Geometry: final body of the model. Coordinates: model frame, mm. Face numbers are marked on the shaded views. A direction names the side the tool comes from. Round coordinates to 2 decimals unless told otherwise and drop trailing zeros. Loops run counter-clockwise (first coordinate to the right, second up) from the corner with the lowest first, then second, coordinate; pieces in that order, holes last. Notation, with made-up numbers: (31, 85) -> (52, 85) arc R21 ccw to (52, 111) -> close; hole circle Ø7 at (71, -23.5). An arc over 180 degrees is marked (long way). Answer in a Markdown table with one row per item.
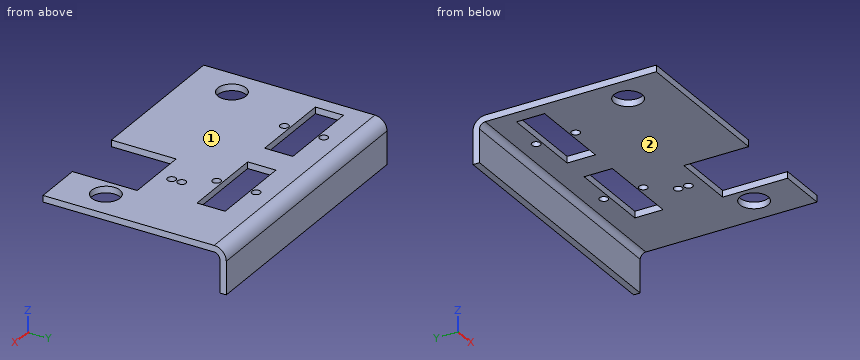
```python
from build123d import *

# Parameters (mm, degrees)
SKETCH1_W                    = 95
SKETCH1_H                    = 65
BASE_FLANGE1_DEPTH           = 2.3
EDGE_FLANGE1_STRIP_W         = 13.2
EDGE_FLANGE1_STRIP_H         = 2.3
EDGE_FLANGE1_STRIP_CUT_DEPTH = 95
EDGE_FLANGE1_DEPTH           = 95
CUT_EXTRUDE1_REACH           = 118.215
SKETCH9_R                    = 1.5
SKETCH9_W                    = 23
SKETCH9_H                    = 23
CUT_EXTRUDE3_REACH           = 117.921
SKETCH10_R                   = 1.5
SKETCH10_W                   = 30
SKETCH10_H                   = 10
CUT_EXTRUDE4_REACH           = 117.921
SKETCH11_R                   = 5


# Sheet-metal steps are written as plain solids
with BuildPart() as part:
    # Sketch1 → Base-Flange1 (new body)
    with BuildSketch(Plane.XY):
        with Locations((47.5, 32.5)):
            Rectangle(SKETCH1_W, SKETCH1_H)
    extrude(amount=-BASE_FLANGE1_DEPTH)

    # Edge-Flange1 strip (across the edge) → Edge-Flange1 strip cut (cut)
    with BuildSketch(Plane(origin=(0, 65, -2.3), x_dir=(0, -1, 0), z_dir=(1, 0, 0))):
        with Locations((-2.3, -1.15)):
            Rectangle(EDGE_FLANGE1_STRIP_W, EDGE_FLANGE1_STRIP_H)
    extrude(amount=EDGE_FLANGE1_STRIP_CUT_DEPTH, mode=Mode.SUBTRACT)

    # Edge-Flange1 section (across the edge) → Edge-Flange1 (add)
    with BuildSketch(Plane(origin=(0, 65, -2.3), x_dir=(0, -1, 0), z_dir=(1, 0, 0))):
        with BuildLine():
            Line((0, 2), (0, 13.7))
            Line((0, 13.7), (2.3, 13.7))
            Line((2.3, 13.7), (2.3, 2))
            ThreePointArc((2.3, 2), (2.885786438, 0.585786438), (4.3, 0))
            Line((4.3, 0), (4.3, -2.3))
            ThreePointArc((4.3, -2.3), (1.259440841, -1.040559159), (0, 2))
        make_face()
    extrude(amount=EDGE_FLANGE1_DEPTH)

    # Sketch9 → Cut-Extrude1 (cut, up to next)
    with BuildSketch(Plane.XY, mode=Mode.PRIVATE) as cut_extrude1_sk1:
        with Locations((66.12, 28.3)):
            Circle(SKETCH9_R)
    cut_extrude1_tool1 = extrude(cut_extrude1_sk1.sketch, amount=-CUT_EXTRUDE1_REACH, mode=Mode.PRIVATE) & part.part
    # Sketch9 → Cut-Extrude1 (cut, up to next)
    with BuildSketch(Plane.XY, mode=Mode.PRIVATE) as cut_extrude1_sk2:
        with Locations((66.12, 31.9)):
            Circle(SKETCH9_R)
    cut_extrude1_tool2 = extrude(cut_extrude1_sk2.sketch, amount=-CUT_EXTRUDE1_REACH, mode=Mode.PRIVATE) & part.part
    # Sketch9 → Cut-Extrude1 (cut, up to next)
    with BuildSketch(Plane.XY, mode=Mode.PRIVATE) as cut_extrude1_sk3:
        with Locations((66.12, 11.5)):
            Rectangle(SKETCH9_W, SKETCH9_H)
    cut_extrude1_tool3 = extrude(cut_extrude1_sk3.sketch, amount=-CUT_EXTRUDE1_REACH, mode=Mode.PRIVATE) & part.part
    add(cut_extrude1_tool1.solids().sort_by_distance((66.12, 28.3, 0))[0], mode=Mode.SUBTRACT)
    add(cut_extrude1_tool2.solids().sort_by_distance((66.12, 31.9, 0))[0], mode=Mode.SUBTRACT)
    add(cut_extrude1_tool3.solids().sort_by_distance((66.12, 11.5, 0))[0], mode=Mode.SUBTRACT)

    # Sketch10 → Cut-Extrude3 (cut, up to next)
    with BuildSketch(Plane(origin=(0, 0, -2.3), x_dir=(-1, 0, 0), z_dir=(0, 0, -1)), mode=Mode.PRIVATE) as cut_extrude3_sk1:
        with Locations((-60, 54.6)):
            Circle(SKETCH10_R)
    cut_extrude3_tool1 = extrude(cut_extrude3_sk1.sketch, amount=-CUT_EXTRUDE3_REACH, mode=Mode.PRIVATE) & part.part
    # Sketch10 → Cut-Extrude3 (cut, up to next)
    with BuildSketch(Plane(origin=(0, 0, -2.3), x_dir=(-1, 0, 0), z_dir=(0, 0, -1)), mode=Mode.PRIVATE) as cut_extrude3_sk2:
        with Locations((-60, 40.6)):
            Circle(SKETCH10_R)
    cut_extrude3_tool2 = extrude(cut_extrude3_sk2.sketch, amount=-CUT_EXTRUDE3_REACH, mode=Mode.PRIVATE) & part.part
    # Sketch10 → Cut-Extrude3 (cut, up to next)
    with BuildSketch(Plane(origin=(0, 0, -2.3), x_dir=(-1, 0, 0), z_dir=(0, 0, -1)), mode=Mode.PRIVATE) as cut_extrude3_sk3:
        with Locations((-20, 54.6)):
            Circle(SKETCH10_R)
    cut_extrude3_tool3 = extrude(cut_extrude3_sk3.sketch, amount=-CUT_EXTRUDE3_REACH, mode=Mode.PRIVATE) & part.part
    # Sketch10 → Cut-Extrude3 (cut, up to next)
    with BuildSketch(Plane(origin=(0, 0, -2.3), x_dir=(-1, 0, 0), z_dir=(0, 0, -1)), mode=Mode.PRIVATE) as cut_extrude3_sk4:
        with Locations((-20, 40.6)):
            Circle(SKETCH10_R)
    cut_extrude3_tool4 = extrude(cut_extrude3_sk4.sketch, amount=-CUT_EXTRUDE3_REACH, mode=Mode.PRIVATE) & part.part
    # Sketch10 → Cut-Extrude3 (cut, up to next)
    with BuildSketch(Plane(origin=(0, 0, -2.3), x_dir=(-1, 0, 0), z_dir=(0, 0, -1)), mode=Mode.PRIVATE) as cut_extrude3_sk5:
        with Locations((-20, 47.6)):
            Rectangle(SKETCH10_W, SKETCH10_H)
    cut_extrude3_tool5 = extrude(cut_extrude3_sk5.sketch, amount=-CUT_EXTRUDE3_REACH, mode=Mode.PRIVATE) & part.part
    # Sketch10 → Cut-Extrude3 (cut, up to next)
    with BuildSketch(Plane(origin=(0, 0, -2.3), x_dir=(-1, 0, 0), z_dir=(0, 0, -1)), mode=Mode.PRIVATE) as cut_extrude3_sk6:
        with Locations((-60, 47.6)):
            Rectangle(SKETCH10_W, SKETCH10_H)
    cut_extrude3_tool6 = extrude(cut_extrude3_sk6.sketch, amount=-CUT_EXTRUDE3_REACH, mode=Mode.PRIVATE) & part.part
    add(cut_extrude3_tool1.solids().sort_by_distance((60, 54.6, -2.3))[0], mode=Mode.SUBTRACT)
    add(cut_extrude3_tool2.solids().sort_by_distance((60, 40.6, -2.3))[0], mode=Mode.SUBTRACT)
    add(cut_extrude3_tool3.solids().sort_by_distance((20, 54.6, -2.3))[0], mode=Mode.SUBTRACT)
    add(cut_extrude3_tool4.solids().sort_by_distance((20, 40.6, -2.3))[0], mode=Mode.SUBTRACT)
    add(cut_extrude3_tool5.solids().sort_by_distance((20, 47.6, -2.3))[0], mode=Mode.SUBTRACT)
    add(cut_extrude3_tool6.solids().sort_by_distance((60, 47.6, -2.3))[0], mode=Mode.SUBTRACT)

    # Sketch11 → Cut-Extrude4 (cut, up to next)
    with BuildSketch(Plane(origin=(0, 0, -2.3), x_dir=(-1, 0, 0), z_dir=(0, 0, -1)), mode=Mode.PRIVATE) as cut_extrude4_sk1:
        with Locations((-10, 16)):
            Circle(SKETCH11_R)
    cut_extrude4_tool1 = extrude(cut_extrude4_sk1.sketch, amount=-CUT_EXTRUDE4_REACH, mode=Mode.PRIVATE) & part.part
    # Sketch11 → Cut-Extrude4 (cut, up to next)
    with BuildSketch(Plane(origin=(0, 0, -2.3), x_dir=(-1, 0, 0), z_dir=(0, 0, -1)), mode=Mode.PRIVATE) as cut_extrude4_sk2:
        with Locations((-84.5, 16)):
            Circle(SKETCH11_R)
    cut_extrude4_tool2 = extrude(cut_extrude4_sk2.sketch, amount=-CUT_EXTRUDE4_REACH, mode=Mode.PRIVATE) & part.part
    add(cut_extrude4_tool1.solids().sort_by_distance((10, 16, -2.3))[0], mode=Mode.SUBTRACT)
    add(cut_extrude4_tool2.solids().sort_by_distance((84.5, 16, -2.3))[0], mode=Mode.SUBTRACT)


solid = part.part
```
Item 1: Section query B-B, the plane y = 54.6. Output: boundary loops of the cut face in (x, z), and give its area (3 significant figures).
Ans:
| item | result |
|---|---|
| outline | (0, -2.3) -> (18.5, -2.3) -> (18.5, 0) -> (0, 0) -> close; (21.5, -2.3) -> (58.5, -2.3) -> (58.5, 0) -> (21.5, 0) -> close; (61.5, -2.3) -> (95, -2.3) -> (95, 0) -> (61.5, 0) -> close |
| area | 205 mm2 |
Item 2: Section query D-D, the plane y = 16. Output: boundary loops of the cut face in (x, z), and give its area (3 significant figures).
Ans:
| item | result |
|---|---|
| outline | (0, -2.3) -> (5, -2.3) -> (5, 0) -> (0, 0) -> close; (15, -2.3) -> (54.62, -2.3) -> (54.62, 0) -> (15, 0) -> close; (77.62, -2.3) -> (79.5, -2.3) -> (79.5, 0) -> (77.62, 0) -> close; (89.5, -2.3) -> (95, -2.3) -> (95, 0) -> (89.5, 0) -> close |
| area | 120 mm2 |
Item 3: First-contact query: P1, Ø3.5, axis at x = 29.5, z = -8.5, coming from the -Y side; P2, Ø8, axis at y = 57, z = -10, coming from the +X side; P3, Ø1.8, axis at x = 62.5, z = -1, coming from the -Y side; P4, Ø1.2, axis at x = 15, z = -1.5, coming from the +Y side. Flat tips, straight axial feed; report the tip coordinate or a pass-through.
Ans:
| item | result |
|---|---|
| P1 | y = 62.7 |
| P2 | through |
| P3 | y = 23 |
| P4 | y = 64.39 |
Item 4: Section query C-C, the plane x = 60. Output: boundary loops of the cut face in (y, z).
Ans:
| item | result |
|---|---|
| outline | (23, -2.3) -> (39.1, -2.3) -> (39.1, 0) -> (23, 0) -> close; (42.1, -2.3) -> (42.6, -2.3) -> (42.6, 0) -> (42.1, 0) -> close; (52.6, -2.3) -> (53.1, -2.3) -> (53.1, 0) -> (52.6, 0) -> close; (56.1, -2.3) -> (60.7, -2.3) arc R2 cw to (62.7, -4.3) -> (62.7, -16) -> (65, -16) -> (65, -4.3) arc R4.3 ccw to (60.7, 0) -> (56.1, 0) -> close |
Item 5: Ray query, L1, parallel to Y at x = 60, z = -1.05; L2, parallel to Y at x = 20, z = -0.6; L3, parallel to Y at x = 27, z = -12.5. Return the intervals inside material, ascending.
Ans:
| item | result |
|---|---|
| L1 | 23 to 39.1, 42.1 to 42.6, 52.6 to 53.1, 56.1 to 63.52 |
| L2 | 0 to 39.1, 42.1 to 42.6, 52.6 to 53.1, 56.1 to 62.89 |
| L3 | 62.7 to 65 |
Item 6: Set-up query: the marked faces 1 and 2. Return all of +Z, -Z, +X, -X, +Y, -Y with unobstructed straight access to the full face (end or side cutting, diameter ignored); none if empty.
Ans:
| item | result |
|---|---|
| face 1 | +Z, +X, -X, +Y, -Y |
| face 2 | -Z, +X, -X, -Y |
Item 7: Section query A-A, the plane x = 87.5. Output: boundary loops of the cut face in (y, z), and give its area (4 significant figures).
Ans:
| item | result |
|---|---|
| outline | (0, -2.3) -> (12, -2.3) -> (12, 0) -> (0, 0) -> close; (20, -2.3) -> (60.7, -2.3) arc R2 cw to (62.7, -4.3) -> (62.7, -16) -> (65, -16) -> (65, -4.3) arc R4.3 ccw to (60.7, 0) -> (20, 0) -> close |
| area | 159.5 mm2 |
